CAD build for the part. Positions are in the model's coordinates, mm. A direction names the side the tool comes from. Coordinates: 2 decimals unless noted, no trailing zeros. Order: outer loops, then holes, each group sorted by start corner. A loop starts at its lowest first (then second) coordinate and runs counter-clockwise, first axis right, second up. Notation, with made-up numbers: (-15, 28) - (18, 28) arc R19 cw to (18, 32) - close; hole circle Ø10 at (65.25, 38). An arc over 180 degrees is marked (long way). Use one line per item in the form item = value.
```python
from build123d import *

# Parameters (mm, degrees)
BOSS_EXTRUDE1_DEPTH            = 10
SKETCH2_R                      = 22.5
CUT_EXTRUDE1_DEPTH             = 112.804516903
SKETCH3_R                      = 2
CUT_EXTRUDE2_DEPTH             = 112.804516903
SKETCH5_W                      = 38
SKETCH5_H                      = 64
BOSS_EXTRUDE2_DEPTH            = 40
SKETCH6_W                      = 20
SKETCH6_H                      = 20
CUT_EXTRUDE3_DEPTH             = 139.290455202
CUT_EXTRUDE4_REACH             = 124.067
SKETCH8_R                      = 2
CUT_EXTRUDE4_DIRECTION_2_DEPTH = 123.066580193
CUT_EXTRUDE5_REACH             = 213.189
SKETCH9_R                      = 2
CUT_EXTRUDE6_REACH             = 213.189
SKETCH10_R                     = 2
FILLET1_R                      = 3
FILLET2_R                      = 3
FILLET3_R                      = 3


with BuildPart() as part:
    # Sketch1 → Boss-Extrude1 (new body)
    with BuildSketch(Plane.XY):
        with BuildLine():
            Line((38.418745425, 32), (99.5, 32))
            Line((99.5, 32), (99.5, -32))
            Line((99.5, -32), (38.418745425, -32))
            ThreePointArc((38.418745425, -32), (0, -50), (-38.418745425, -32))
            Line((-38.418745425, -32), (-99.5, -32))
            Line((-99.5, -32), (-99.5, 32))
            Line((-99.5, 32), (-38.418745425, 32))
            ThreePointArc((-38.418745425, 32), (0, 50), (38.418745425, 32))
        make_face()
    extrude(amount=BOSS_EXTRUDE1_DEPTH)

    # Sketch2 → Cut-Extrude1 (cut, through all)
    with BuildSketch(Plane.XY.offset(10)):
        Circle(SKETCH2_R)
    extrude(amount=-CUT_EXTRUDE1_DEPTH, mode=Mode.SUBTRACT)

    # Sketch3 → Cut-Extrude2 (cut, through all)
    with BuildSketch(Plane.XY.offset(10)):
        with Locations((32, 0)):
            Circle(SKETCH3_R)
        with Locations((22.627416998, -22.627416998)):
            Circle(SKETCH3_R)
        with Locations((0, -32)):
            Circle(SKETCH3_R)
        with Locations((-22.627416998, -22.627416998)):
            Circle(SKETCH3_R)
        with Locations((-32, 0)):
            Circle(SKETCH3_R)
        with Locations((-22.627416998, 22.627416998)):
            Circle(SKETCH3_R)
        with Locations((0, 32)):
            Circle(SKETCH3_R)
        with Locations((22.627416998, 22.627416998)):
            Circle(SKETCH3_R)
    extrude(amount=-CUT_EXTRUDE2_DEPTH, mode=Mode.SUBTRACT)

    # Sketch5 → Boss-Extrude2 (add)
    with BuildSketch(Plane.XY.offset(10)):
        with Locations((80.5, 0)):
            Rectangle(SKETCH5_W, SKETCH5_H)
        with Locations((-80.5, 0)):
            Rectangle(SKETCH5_W, SKETCH5_H)
    extrude(amount=BOSS_EXTRUDE2_DEPTH)

    # Sketch6 → Cut-Extrude3 (cut, through all)
    with BuildSketch(Plane(origin=(0, 32, 0), x_dir=(1, 0, 0), z_dir=(0, 1, 0))):
        with Locations((80.5, -30)):
            Rectangle(SKETCH6_W, SKETCH6_H)
        with Locations((-80.5, -30)):
            Rectangle(SKETCH6_W, SKETCH6_H)
    extrude(amount=-CUT_EXTRUDE3_DEPTH, mode=Mode.SUBTRACT)

    # Sketch8 → Cut-Extrude4 (cut, up to next)
    with BuildSketch(Plane.XY.offset(50), mode=Mode.PRIVATE) as cut_extrude4_sk1:
        with Locations(Location((80.5, 14, 0), (0, 0, 180))):
            Circle(SKETCH8_R)
    cut_extrude4_tool1 = extrude(cut_extrude4_sk1.sketch, amount=-CUT_EXTRUDE4_REACH, mode=Mode.PRIVATE) & part.part
    # Sketch8 → Cut-Extrude4 (cut, up to next)
    with BuildSketch(Plane.XY.offset(50), mode=Mode.PRIVATE) as cut_extrude4_sk2:
        with Locations(Location((80.5, -14, 0), (0, 0, 180))):
            Circle(SKETCH8_R)
    cut_extrude4_tool2 = extrude(cut_extrude4_sk2.sketch, amount=-CUT_EXTRUDE4_REACH, mode=Mode.PRIVATE) & part.part
    # Sketch8 → Cut-Extrude4 (cut, up to next)
    with BuildSketch(Plane.XY.offset(50), mode=Mode.PRIVATE) as cut_extrude4_sk3:
        with Locations(Location((-80.5, -14, 0), (0, 0, 180))):
            Circle(SKETCH8_R)
    cut_extrude4_tool3 = extrude(cut_extrude4_sk3.sketch, amount=-CUT_EXTRUDE4_REACH, mode=Mode.PRIVATE) & part.part
    # Sketch8 → Cut-Extrude4 (cut, up to next)
    with BuildSketch(Plane.XY.offset(50), mode=Mode.PRIVATE) as cut_extrude4_sk4:
        with Locations(Location((-80.5, 14, 0), (0, 0, 180))):
            Circle(SKETCH8_R)
    cut_extrude4_tool4 = extrude(cut_extrude4_sk4.sketch, amount=-CUT_EXTRUDE4_REACH, mode=Mode.PRIVATE) & part.part
    add(cut_extrude4_tool1.solids().sort_by_distance((80.5, 14, 50))[0], mode=Mode.SUBTRACT)
    add(cut_extrude4_tool2.solids().sort_by_distance((80.5, -14, 50))[0], mode=Mode.SUBTRACT)
    add(cut_extrude4_tool3.solids().sort_by_distance((-80.5, -14, 50))[0], mode=Mode.SUBTRACT)
    add(cut_extrude4_tool4.solids().sort_by_distance((-80.5, 14, 50))[0], mode=Mode.SUBTRACT)

    # Sketch8 → Cut-Extrude4 direction 2 (cut)
    with BuildSketch(Plane.XY.offset(50)):
        with Locations(Location((80.5, 14, 0), (0, 0, 180))):
            Circle(SKETCH8_R)
        with Locations(Location((80.5, -14, 0), (0, 0, 180))):
            Circle(SKETCH8_R)
        with Locations(Location((-80.5, -14, 0), (0, 0, 180))):
            Circle(SKETCH8_R)
        with Locations(Location((-80.5, 14, 0), (0, 0, 180))):
            Circle(SKETCH8_R)
    extrude(amount=CUT_EXTRUDE4_DIRECTION_2_DEPTH, mode=Mode.SUBTRACT)

    # Sketch9 → Cut-Extrude5 (cut, up to next)
    with BuildSketch(Plane(origin=(99.5, 0, 0), x_dir=(0, 0, -1), z_dir=(1, 0, 0)), mode=Mode.PRIVATE) as cut_extrude5_sk1:
        with Locations((-30, 14)):
            Circle(SKETCH9_R)
    cut_extrude5_tool1 = extrude(cut_extrude5_sk1.sketch, amount=-CUT_EXTRUDE5_REACH, mode=Mode.PRIVATE) & part.part
    # Sketch9 → Cut-Extrude5 (cut, up to next)
    with BuildSketch(Plane(origin=(99.5, 0, 0), x_dir=(0, 0, -1), z_dir=(1, 0, 0)), mode=Mode.PRIVATE) as cut_extrude5_sk2:
        with Locations((-30, -14)):
            Circle(SKETCH9_R)
    cut_extrude5_tool2 = extrude(cut_extrude5_sk2.sketch, amount=-CUT_EXTRUDE5_REACH, mode=Mode.PRIVATE) & part.part
    add(cut_extrude5_tool1.solids().sort_by_distance((99.5, 14, 30))[0], mode=Mode.SUBTRACT)
    add(cut_extrude5_tool2.solids().sort_by_distance((99.5, -14, 30))[0], mode=Mode.SUBTRACT)

    # Sketch10 → Cut-Extrude6 (cut, up to next)
    with BuildSketch(Plane.ZY.offset(99.5), mode=Mode.PRIVATE) as cut_extrude6_sk1:
        with Locations(Location((30, 14, 0), (0, 0, 180))):
            Circle(SKETCH10_R)
    cut_extrude6_tool1 = extrude(cut_extrude6_sk1.sketch, amount=-CUT_EXTRUDE6_REACH, mode=Mode.PRIVATE) & part.part
    # Sketch10 → Cut-Extrude6 (cut, up to next)
    with BuildSketch(Plane.ZY.offset(99.5), mode=Mode.PRIVATE) as cut_extrude6_sk2:
        with Locations(Location((30, -14, 0), (0, 0, 180))):
            Circle(SKETCH10_R)
    cut_extrude6_tool2 = extrude(cut_extrude6_sk2.sketch, amount=-CUT_EXTRUDE6_REACH, mode=Mode.PRIVATE) & part.part
    add(cut_extrude6_tool1.solids().sort_by_distance((-99.5, 14, 30))[0], mode=Mode.SUBTRACT)
    add(cut_extrude6_tool2.solids().sort_by_distance((-99.5, -14, 30))[0], mode=Mode.SUBTRACT)

    # Fillet1
    fillet1_edges = [part.edges().sort_by_distance(p)[0] for p in [
        (61.5, 0, 10),
        (-61.5, 0, 10),
    ]]
    fillet(fillet1_edges, radius=FILLET1_R)

    # Fillet2
    fillet2_edges = [part.edges().sort_by_distance(p)[0] for p in [
        (99.5, 0, 50),
        (61.5, 0, 50),
        (-61.5, 0, 50),
        (-99.5, 0, 50),
    ]]
    fillet(fillet2_edges, radius=FILLET2_R)

    # Fillet3
    fillet3_edges = [part.edges().sort_by_distance(p)[0] for p in [
        (99.5, 0, 0),
        (-99.5, 0, 0),
    ]]
    fillet(fillet3_edges, radius=FILLET3_R)


solid = part.part
```
Item 1: Two-plate mould, pull along X, no slides. Class faces 1 (the face through (-70.5, 0, 30)), 2 (the face through (-0.613, 49.996, 4.93)), 3 (the face through (-99.5, 0, 25)), 4 (the face through (-75, -32, 19)): +X half, -X half, draft (parallel to the pull), parting line (faces both ways), or undercut.
Derived:
face_1 = undercut
face_2 = parting line
face_3 = -X half
face_4 = draft
Item 2: Cut at B-B, the plane z = 30. State how many separate pieces and enclosed holes the cut face has, plus the area to 3 significant figures.
Derived:
separate_pieces = 8
enclosed_holes = 0
area = 2,160 mm²
Item 3: Cut at C-C, the plane y = 4. Write the cut outline in (x, z).
Derived:
outline = (-99.5, 3) arc R3 ccw to (-96.5, 0) - (-22.14, 0) - (-22.14, 10) - (-58.5, 10) arc R3 cw to (-61.5, 13) - (-61.5, 47) arc R3 ccw to (-64.5, 50) - (-96.5, 50) arc R3 ccw to (-99.5, 47) - close; (22.14, 0) - (96.5, 0) arc R3 ccw to (99.5, 3) - (99.5, 47) arc R3 ccw to (96.5, 50) - (64.5, 50) arc R3 ccw to (61.5, 47) - (61.5, 13) arc R3 cw to (58.5, 10) - (22.14, 10) - close; hole (-90.5, 20) - (-70.5, 20) - (-70.5, 40) - (-90.5, 40) - close; hole (70.5, 20) - (90.5, 20) - (90.5, 40) - (70.5, 40) - close
Item 4: Drop flat-ended pins along their axis: pin 1 (5 mm diameter, centred on x = -32, y = 0, fed in from +Z); pin 2 (2 mm diameter, centred on x = -44, y = -33.5, fed in from -Z); pin 3 (2.5 mm diameter, centred on y = 14, z = 30, fed in from -X). Give the stop position or say it passes through.
Derived:
pin_1 = 10
pin_2 = through
pin_3 = -70.5
Item 5: Cut at D-D, the plane x = 80.5. Write the cut outline in (y, z).
Derived:
outline = (-32, 0) - (32, 0) - (32, 20) - (-32, 20) - close; (-32, 40) - (-16, 40) - (-16, 50) - (-32, 50) - close; (-12, 40) - (12, 40) - (12, 50) - (-12, 50) - close; (16, 40) - (32, 40) - (32, 50) - (16, 50) - close
Item 6: Cut at A-A, the plane x = 32. Write the cut outline in (y, z), plus the area to 3 significant figures.
Derived:
outline = (-38.42, 0) - (-2, 0) - (-2, 10) - (-38.42, 10) - close; (2, 0) - (38.42, 0) - (38.42, 10) - (2, 10) - close
area = 728 mm²
Item 7: 3-axis set-ups, long thin cutter, end or side, ignore diameter. For faces 5 (the face through (-90.5, 0, 30)), 6 (the face through (-76, 32, 19)), 7 (the face through (61.5, 0, 30)): which of +Z, -Z, +X, -X, +Y, -Y reach the whole face in a straight line?
Derived:
face_5 = +Y, -Y
face_6 = +Z, -Z, -X, +Y
face_7 = +Z, +Y, -Y
Item 8: Drill centre lines: line 1 (X direction, y = -7, z = 28.5); line 2 (Y direction, x = 93.25, z = 30); line 3 (Z direction, x = 74, y = -22.5). Where is each one in solid material? Low to high. Write a range as [from, to].
Derived:
line_1 = [-99.5, -90.5], [-70.5, -61.5], [61.5, 70.5], [90.5, 99.5]
line_2 = [-32, -16], [-12, 12], [16, 32]
line_3 = [0, 20], [40, 50]
